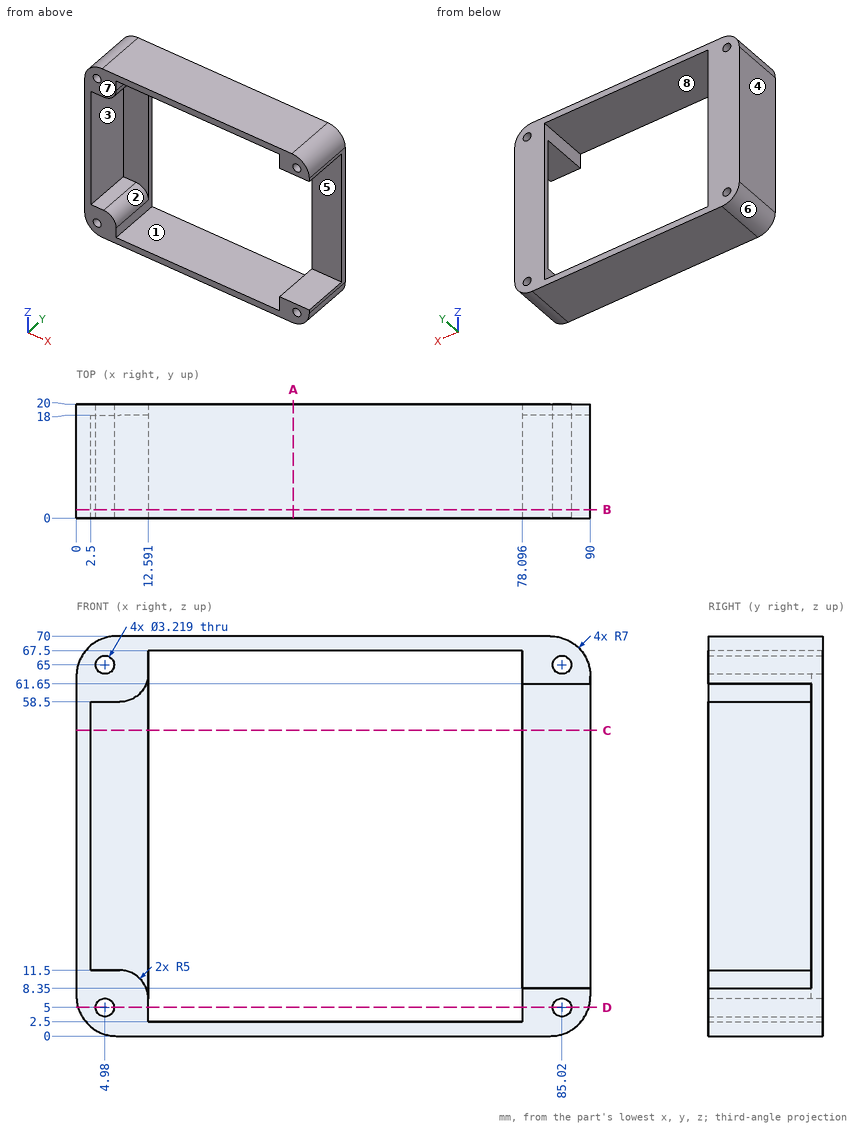
Design review of the part shown in the three views and the two pictorial views. Dimensions are in mm from the part's minimum x, y and z. A direction names the side the tool comes from. Round coordinates to 2 decimals unless told otherwise and drop trailing zeros. Write each loop counter-clockwise with the first axis right and the second up, starting at its lowest first coordinate (ties: lowest second). Pieces come first, ordered by that corner, then holes.
Item 1: For pin 1 Ø5.5 at (y, z) = (8, 24.5) entering from +X; pin 2 Ø3.5 at (x, y) = (86.5, 8.5) entering from -Z; pin 3 Ø3 at (x, z) = (8, 34) entering from -Y, all flat-tipped, find the tip position at first contact; note any pin that passes through.
Item 2: Consider section C-C on z = 53.5. Give the boundary of the cut face in (x, y).
Item 3: For the marked faces 1, 2, 3 and 4, list the 3-axis set-ups (+Z, -Z, +X, -X, +Y, -Y) from which the entire face can be reached by the end or side of a thin tool; tool diameter is ignored.
Item 4: Wall thickness on L1, parallel to Z at x = 35.5, y = 3.5; L2, parallel to X at y = 11, z = 5; L3, parallel to X at y = 1.5, z = 65.5: over which ranges is each line inside the solid? List them lowest first.
Item 5: Consider section B-B on y = 1.5. Give the boundary of the cut face in (x, z).
Item 6: Consider section D-D on z = 5. Give the boundary of the cut face in (x, y).
Item 7: Consider section A-A on x = 38. Give the boundary of the cut face in (y, z), and give its area (3 significant figures).
Item 8: Draft analysis for pull direction Z (two halves, no side actions). For the marked faces 5, 6, 7 and 8, state which applies: released by +Z, released by -Z, zero draft, split by the parting line, or undercut.
Check values:
1. pin 1: stops at x = 2.5
1. pin 2: stops at z = 0.22
1. pin 3: stops at y = 18
2. outline: (0, 0) - (2.5, 0) - (2.5, 18) - (12.59, 18) - (12.59, 20) - (0, 20) - close; (78.1, 18) - (90, 18) - (90, 20) - (78.1, 20) - close
3. face 1: +Y, -Y
3. face 2: -Y
3. face 3: +X, -Y
3. face 4: +Z, -Z, -X, +Y, -Y
4. L1: z = 0 to 2.5, 67.5 to 70
4. L2: x = 0.29 to 3.37, 6.59 to 12.59, 78.1 to 83.41, 86.63 to 89.71
4. L3: x = 0.46 to 3.45, 6.51 to 12.59, 78.1 to 83.49, 86.55 to 89.54
5. outline: (0, 7) arc R7 ccw to (7, 0) - (83, 0) arc R7 ccw to (90, 7) - (90, 8.35) - (78.1, 8.35) - (78.1, 2.5) - (12.59, 2.5) - (12.59, 6.5) arc R5 ccw to (7.59, 11.5) - (2.5, 11.5) - (2.5, 58.5) - (7.59, 58.5) arc R5 ccw to (12.59, 63.5) - (12.59, 67.5) - (78.1, 67.5) - (78.1, 61.65) - (90, 61.65) - (90, 63) arc R7 ccw to (83, 70) - (7, 70) arc R7 ccw to (0, 63) - close; hole circle Ø3.22 at (4.98, 5); hole circle Ø3.22 at (4.98, 65); hole circle Ø3.22 at (85.02, 5); hole circle Ø3.22 at (85.02, 65)
6. outline: (0.29, 0) - (3.37, 0) - (3.37, 20) - (0.29, 20) - close; (6.59, 0) - (12.59, 0) - (12.59, 20) - (6.59, 20) - close; (78.1, 0) - (83.41, 0) - (83.41, 20) - (78.1, 20) - close; (86.63, 0) - (89.71, 0) - (89.71, 20) - (86.63, 20) - close
7. outline: (0, 0) - (20, 0) - (20, 2.5) - (0, 2.5) - close; (0, 67.5) - (20, 67.5) - (20, 70) - (0, 70) - close
7. area: 100 mm2
8. face 5: undercut
8. face 6: released by -Z
8. face 7: zero draft
8. face 8: undercut
